Design review of the part built by this model. Coordinates are the model's own, in mm. Coordinates: 2 decimals unless noted, no trailing zeros. Write each loop counter-clockwise with the first axis right and the second up, starting at its lowest first coordinate (ties: lowest second). Pieces come first, ordered by that corner, then holes. Notation, with made-up numbers: (11.25, 72) - (16.25, 72) arc R18 ccw to (16.25, 87) - close; hole circle Ø2 at (-8.75, 66.25). An arc over 180 degrees is marked (long way). Use a Markdown table: item, result.
Autodesk Fusion 360 part; units mm, degrees
sketch "LightResistorMeasurement" plane through (0, 0, 0) normal (0, 0, 1) x (1, 0, 0)
  line L0 (0, 0) -> (0.0874, 0)
  line L1 (0, 0) -> (0, 2) construction
  line L2 (0, 0) -> (0, -2) construction
  line L3 (0, 2) -> (1.5, 2)
  line L4 (0, 2) -> (-1.5, 2)
  line L5 (0, -2) -> (1.5, -2)
  line L6 (0, -2) -> (-1.5, -2)
  arc A0 (-1.5, 2) -> (-1.5, -2) centre (0, 0) ccw
  arc A1 (1.5, -2) -> (1.5, 2) centre (0, 0) ccw
  line L7 (0, 0) -> (2, 0) construction
  line L8 (0, 0) -> (-2, 0) construction
  circle A2 centre (-1.7, 0) radius 0.3
  circle A3 centre (1.7, 0) radius 0.3
  dimension "d1" = 5
  dimension "d2" = 2
  dimension "d3" = 2
  dimension "d4" = 2
  dimension "d5" = 0.6
  dimension "d6" = 0.6
extrude "Extrude1" add sketch "LightResistorMeasurement" along normal blind 1.8 contours L3 L4 L5 L6 A0 A1 | A2 | A3
extrude "Extrude2" add sketch "LightResistorMeasurement" against normal blind 24 contours A2 | A3
extrude "Extrude3" add sketch "LightResistorMeasurement" along normal blind 2 contours A2 | A3
(1) Take a section at C-C on x = 1.75. Write out the cut boundary in (y, z), and give its area (3 significant figures).
Determined:
| item | result |
|---|---|
| outline | (-1.79, 0) - (-0.3, 0) - (-0.3, -24) - (0.3, -24) - (0.3, 0) - (1.79, 0) - (1.79, 1.8) - (0.3, 1.8) - (0.3, 2) - (-0.3, 2) - (-0.3, 1.8) - (-1.79, 1.8) - close |
| area | 20.7 mm2 |
(2) Take a section at A-A on y = 0. Write out the cut boundary in (x, z), and give its area (3 significant figures).
Determined:
| item | result |
|---|---|
| outline | (-2.5, 0) - (-2, 0) - (-2, -24) - (-1.4, -24) - (-1.4, 0) - (1.4, 0) - (1.4, -24) - (2, -24) - (2, 0) - (2.5, 0) - (2.5, 1.8) - (2, 1.8) - (2, 2) - (1.4, 2) - (1.4, 1.8) - (-1.4, 1.8) - (-1.4, 2) - (-2, 2) - (-2, 1.8) - (-2.5, 1.8) - close |
| area | 38.0 mm2 |
(3) For L1, parallel to Z at x = -1.7, y = -1.8; L2, parallel to X at y = -0.15, z = -9.25; L3, parallel to X at y = 0.25, z = -9, list the stretches that pass through material, from the lowest coordinate up. Write a range as from..to.
Determined:
| item | result |
|---|---|
| L1 | 0..1.8 |
| L2 | -1.96..-1.44, 1.44..1.96 |
| L3 | -1.87..-1.53, 1.53..1.87 |
(4) Take a section at D-D on y = 1.5. Write out the cut boundary in (x, z), and give its area (3 significant figures).
Determined:
| item | result |
|---|---|
| outline | (-2, 0) - (2, 0) - (2, 1.8) - (-2, 1.8) - close |
| area | 7.20 mm2 |
(5) Take a section at B-B on z = -15.5. Write out the cut boundary in (x, y), and give its area (3 significant figures).
Determined:
| item | result |
|---|---|
| outline | circle Ø0.6 at (-1.7, 0); circle Ø0.6 at (1.7, 0) |
| area | 0.565 mm2 |
(6) For pin 1 (1.5 mm diameter, centred on x = -2, z = -5, fed in from -Y); pin 2 (2 mm diameter, centred on x = 0, y = 0, fed in from +Z), all flat-tipped, find the tip position at first contact; note any pin that passes through.
Determined:
| item | result |
|---|---|
| pin 1 | y = -0.3 |
| pin 2 | z = 1.8 |
